```python
from build123d import *

# Parameters (mm, degrees)
BOX008_W          = 12.75
BOX008_H          = 3.25
BOX008_DEPTH      = 14
CYLINDER004_R     = 6.375
CYLINDER004_DEPTH = 3.25
CYLINDER002_R     = 6.375
CYLINDER002_DEPTH = 3.25
BOX009_W          = 40.25
BOX009_H          = 3.25
BOX009_DEPTH      = 26
BOX007_W          = 40.25
BOX007_H          = 44
BOX007_DEPTH      = 3.25
CYLINDER003_R     = 20.12
CYLINDER003_DEPTH = 3.25
FILLET008_1_R     = 2
FILLET008_2_R     = 1


with BuildPart() as cube004:
    # Box008 → Box008 (new body)
    with BuildSketch(Plane(origin=(13.75, 40.75, 18), x_dir=(1, 0, 0), z_dir=(0, 0, 1))):
        with Locations((6.375, 1.625)):
            Rectangle(BOX008_W, BOX008_H)
    extrude(amount=BOX008_DEPTH)


with BuildPart() as cylinder004:
    # Cylinder004 → Cylinder004 (new body)
    with BuildSketch(Plane(origin=(20.12, 44, 17.75), x_dir=(1, 0, 0), z_dir=(0, -1, 0))):
        Circle(CYLINDER004_R)
    extrude(amount=CYLINDER004_DEPTH)


with BuildPart() as cylinder002:
    # Cylinder002 → Cylinder002 (new body)
    with BuildSketch(Plane(origin=(20.12, 44, 31.75), x_dir=(1, 0, 0), z_dir=(0, -1, 0))):
        Circle(CYLINDER002_R)
    extrude(amount=CYLINDER002_DEPTH)


with BuildPart() as cube005:
    # Box009 → Box009 (new body)
    with BuildSketch(Plane(origin=(0, 40.75, 0), x_dir=(1, 0, 0), z_dir=(0, 0, 1))):
        with Locations((20.125, 1.625)):
            Rectangle(BOX009_W, BOX009_H)
    extrude(amount=BOX009_DEPTH)


with BuildPart() as fusion:
    # Box007 → Box007 (new body)
    with BuildSketch(Plane.XY):
        with Locations((20.125, 22)):
            Rectangle(BOX007_W, BOX007_H)
    extrude(amount=BOX007_DEPTH)

    # Fusion: union Cube005
    add(cube005.part)


with BuildPart() as fillet008:
    # Cylinder003 → Cylinder003 (new body)
    with BuildSketch(Plane(origin=(20.12, 44, 26.25), x_dir=(1, 0, 0), z_dir=(0, -1, 0))):
        Circle(CYLINDER003_R)
    extrude(amount=CYLINDER003_DEPTH)

    # Fusion001: union Fusion
    add(fusion.part)

    # Cut: cut Cylinder002
    add(cylinder002.part, mode=Mode.SUBTRACT)

    # Cut001: cut Cylinder004
    add(cylinder004.part, mode=Mode.SUBTRACT)

    # Cut002: cut Cube004
    add(cube004.part, mode=Mode.SUBTRACT)

    # Fillet008 1
    fillet008_1_edges = [fillet008.edges().sort_by_distance(p)[0] for p in [
        (20.125, 44, 0),
        (40.25, 0, 1.625),
        (0, 0, 1.625),
    ]]
    fillet(fillet008_1_edges, radius=FILLET008_1_R)

    # Fillet008 2
    fillet008_2_edges = [fillet008.edges().sort_by_distance(p)[0] for p in [
        (20.125, 40.75, 3.25),
    ]]
    fillet(fillet008_2_edges, radius=FILLET008_2_R)


solid = fillet008.part
```
Design review of the part built by this model. Coordinates are the model's own, in mm. A direction names the side the tool comes from. Coordinates: 2 decimals unless noted, no trailing zeros. Write each loop counter-clockwise with the first axis right and the second up, starting at its lowest first coordinate (ties: lowest second). Pieces come first, ordered by that corner, then holes.
1) Add section A-A (z = 19). Write out the cut boundary in (x, y).
2) Add section B-B (x = 20.12). Write out the cut boundary in (y, z) (3 decimals), plus the area to 3 significant figures.
3) To check wall thickness, follow L1, parallel to Z at x = 36.5, y = 3; L2, parallel to Y at x = 15, z = 12.5; L3, parallel to X at y = 41.5, z = 42. State the ranges of each line that lie inside material, in increasing order.
4) Mouldability with a two-part tool opening along X and no side actions: class faces 4 (the flat face through (20, 0, 2)), 5 (the flat face through (0, 31, 2)), 6 (the cylindrical face through (20.009, 42.398, 38.124)) as +X half, -X half, draft (parallel to the pull), parting line (faces both ways), or undercut.
5) Add section C-C (x = 9). Write out the cut boundary in (y, z).
6) Add section D-D (y = 28.5). Write out the cut boundary in (x, z), plus the area to 3 significant figures.
7) Insertion check: pin 1 (1.6 mm diameter, centred on y = 42.5, z = 28, fed in from -X); pin 2 (4 mm diameter, centred on x = 16.5, z = 25, fed in from +Y); pin 3 (1.5 mm diameter, centred on x = 29.5, z = 19.5, fed in from -Y); pin 4 (1.5 mm diameter, centred on x = 33.5, y = 17.5, fed in from +Z). Each pin has a flat end and moves straight along its axis. Give the tip position at first contact, or say it passes through.
8) Machinability: for faces 1 (the cylindrical face through (19.975, 42.398, 11.377)), 2 (the flat face through (11, 40.75, 25)), 3 (the flat face through (29, 44, 24)), which of the approach directions +Z, -Z, +X, -X, +Y, -Y give a long, thin tool a straight path to every point of the face, cutting with its end or side? Answer none if there is none.
Check result:
1. outline: (0, 40.75) - (13.75, 40.75) - (13.75, 44) - (0, 44) - close; (26.5, 40.75) - (40.25, 40.75) - (40.25, 44) - (26.5, 44) - close
2. outline: (0, 0) - (42, 0) arc R2 ccw to (44, 2) - (44, 11.375) - (40.75, 11.375) - (40.75, 4.25) arc R1 cw to (39.75, 3.25) - (0, 3.25) - close; (40.75, 38.125) - (44, 38.125) - (44, 46.37) - (40.75, 46.37) - close
2. area: 196 mm2
3. L1: z = 0 to 3.25
3. L2: y = 40.75 to 44
3. L3: x = 7.6 to 32.64
4. face 4: draft
4. face 5: -X half
4. face 6: undercut
5. outline: (0, 0) - (42, 0) arc R2 ccw to (44, 2) - (44, 43.02) - (40.75, 43.02) - (40.75, 4.25) arc R1 cw to (39.75, 3.25) - (0, 3.25) - close
6. outline: (0, 0) - (40.25, 0) - (40.25, 3.25) - (0, 3.25) - close
6. area: 131 mm2
7. pin 1: stops at x = 0.02
7. pin 2: passes through
7. pin 3: stops at y = 40.75
7. pin 4: stops at z = 3.25
8. face 1: +Y, -Y
8. face 2: +Z, +X, -X, -Y
8. face 3: +Z, -Z, +X, -X, +Y
